from build123d import *

# Parameters (mm, degrees)
PAD_DEPTH          = 3
POCKET_DEPTH       = 3.001
FILLET_R           = 1.5
PAD001_DEPTH       = 8.5
SKETCH004_R        = 2
POCKET001_DEPTH    = 11.501
POCKET002_DEPTH    = 8.5
SKETCH007_R        = 1.5
PAD002_DEPTH       = 2
FILLET001_R        = 1
FILLET002_R        = 2
POLARPATTERN_COUNT = 4


with BuildPart() as part:
    # Sketch → Pad (new body)
    with BuildSketch(Plane.XY):
        with BuildLine():
            Line((0, 0), (28, 0))
            ThreePointArc((23.302356, -15.524181), (26.799869, -8.109687), (28, 0))
            Line((23.302356, -15.524181), (30.833474, -23.0553))
            ThreePointArc((23.0553, -30.833474), (27.223611, -27.223611), (30.833474, -23.0553))
            Line((23.0553, -30.833474), (15.524181, -23.302356))
            ThreePointArc((0, -28), (8.109687, -26.799869), (15.524181, -23.302356))
            Line((0, -28), (0, 0))
        make_face()
    extrude(amount=PAD_DEPTH)

    # Sketch002 (on Face9 of Pad) → Pocket (cut, through all)
    with BuildSketch(Plane.XY.offset(3)):
        Polygon((0, 0), (0, -20), (15.5, -20), (15.5, -15.5), (20, -15.5), (20, 0), align=None)
    extrude(amount=-POCKET_DEPTH, mode=Mode.SUBTRACT)

    # Fillet
    fillet_edges = [part.edges().sort_by_distance(p)[0] for p in [
        (15.5, -15.5, 1.5),
    ]]
    fillet(fillet_edges, radius=FILLET_R)

    # Sketch003 (on Face14 of Fillet) → Pad001 (join)
    with BuildSketch(Plane.XY.offset(3)):
        with BuildLine():
            Line((16.244839, -24.023014), (23.0553, -30.833474))
            ThreePointArc((23.0553, -30.833474), (27.223611, -27.223611), (30.833474, -23.0553))
            Line((30.833474, -23.0553), (24.023014, -16.244839))
            ThreePointArc((16.244839, -24.023014), (20.506097, -20.506097), (24.023014, -16.244839))
        make_face()
    extrude(amount=PAD001_DEPTH)

    # Sketch004 (on Face13 of Pad001) → Pocket001 (cut, through all)
    with BuildSketch(Plane.XY.offset(11.5)):
        with Locations((23.334524, -23.334524)):
            Circle(SKETCH004_R)
    extrude(amount=-POCKET001_DEPTH, mode=Mode.SUBTRACT)

    # Sketch005 (on Face1 of Pocket001) → Pocket002 (cut)
    with BuildSketch(Plane(origin=(0, 0, 0), x_dir=(1, 0, 0), z_dir=(0, 0, -1))):
        with BuildLine():
            ThreePointArc((29.262157, 25.019516), (27.223611, 27.223611), (25.019516, 29.262157))
            Line((25.019516, 29.262157), (18.985551, 23.228191))
            ThreePointArc((23.228191, 18.985551), (21.213203, 21.213203), (18.985551, 23.228191))
            Line((23.228191, 18.985551), (29.262157, 25.019516))
        make_face()
    extrude(amount=-POCKET002_DEPTH, mode=Mode.SUBTRACT)

    # Sketch006 → Groove (revolve, cut)
    with BuildSketch(Plane.YZ):
        Polygon((-38.5, 0), (-38.5, 8.5), (-33, 0), align=None)
    revolve(axis=Axis((0, 0, 0), (0, 0, 1)), mode=Mode.SUBTRACT)

    # Sketch007 (on Face18 of Groove) → Pad002 (join)
    with BuildSketch(Plane.XY.offset(3)):
        with Locations((17, -17)):
            Circle(SKETCH007_R)
    extrude(amount=PAD002_DEPTH)

    # Fillet001
    fillet001_edges = [part.edges().sort_by_distance(p)[0] for p in [
        (20, -15.5, 1.5),
        (15.5, -20, 1.5),
        (18.985551, -23.228191, 4.25),
        (23.228191, -18.985551, 4.25),
    ]]
    fillet(fillet001_edges, radius=FILLET001_R)

    # Fillet002
    fillet002_edges = [part.edges().sort_by_distance(p)[0] for p in [
        (30.833474, -23.0553, 10),
        (23.0553, -30.833474, 10),
    ]]
    fillet(fillet002_edges, radius=FILLET002_R)

    # PolarPattern: part ×4 about axis
    polarpattern_axis = Axis((0, 0, 0), (0, 0, 1))


with BuildPart() as part_1:
    add(part.part)
    for i in range(1, POLARPATTERN_COUNT):
        add(part.part.rotate(polarpattern_axis, i * 360 / POLARPATTERN_COUNT))


solid = part_1.part
For this review, take the finished solid that the model builds, in its own axes (mm). A direction names the side the tool comes from. Coordinates: 2 decimals unless noted, no trailing zeros. Order: outer loops, then holes, each group sorted by start corner. A loop starts at its lowest first (then second) coordinate and runs counter-clockwise, first axis right, second up. Notation, with made-up numbers: (59.25, 10.5) - (88.25, 10.5) arc R31 ccw to (88.25, 37.5) - close; hole circle Ø8 at (20.5, 48.25). An arc over 180 degrees is marked (long way). Answer as CSV lines item,"result". Start each with the question number.
1) To check wall thickness, follow line 1 along Y through (x, z) = (24, 9.5); line 2 along Y through (x, z) = (-21, 1); line 3 along X through (y, z) = (-22.5, 10). State the ranges of each line that lie inside material, in increasing order. Write a range as [from, to].
2) Add section B-B (y = 9). State the section outline as (x, z) points.
3) Add section A-A (z = 9.75). State the section outline as (x, y) points.
4) Draft analysis for pull direction X (two halves, no side actions). For faces 1 (the cylindrical face through (-15.89, 15.99, 3.02)), 2 (the conical face through (27.95, 22.23, 4.19)), 3 (the cylindrical face through (-30.116, 22.775, 9.319)), state which applies: +X half, -X half, draft (parallel to the pull), parting line (faces both ways), or undercut.
5) Add section C-C (x = 2). State the section outline as (y, z) points, then the cut area to 3 significant figures.
6) Machinability: for faces 4 (the flat face through (20, 0, 2)), 5 (the cylindrical face through (21.232, -21.194, 4.19)), 6 (the conical face through (28.14, -21.99, 4.19)), 7 (the cylindrical face through (-27.26, -27.19, 9.98)), 8 (the cylindrical face through (15.99, 15.89, 3.02)), which of the approach directions +Z, -Z, +X, -X, +Y, -Y give a long, thin tool a straight path to every point of the face, cutting with its end or side? Answer none if there is none.
7) Insertion check: P1, Ø2, axis at x = 2, z = 2, coming from the -Y side; P2, Ø0.6, axis at x = -17.5, z = 1, coming from the -Y side; P3, Ø3.5, axis at x = -16.5, y = -16.5, coming from the +Z side; P4, Ø2.5, axis at x = 23.33, y = 23.33, coming from the -Z side. Each pin has a flat end and moves straight along its axis. Give the tip position at first contact, or say it passes through.
Result:
1,line 1,"[-30.01, -25.22], [-21.45, -16.28], [16.28, 21.45], [25.22, 30.01]"
1,line 2,"[-26.29, -25.24], [-21.42, 21.42], [25.24, 26.29]"
1,line 3,"[-30.03, -25.15], [-21.52, -18.3], [18.3, 21.52], [25.15, 30.03]"
2,outline,"(-26.51, 0) - (-20, 0) - (-20, 3) - (-26.51, 3) - close; (20, 0) - (26.51, 0) - (26.51, 3) - (20, 3) - close"
3,outline,"(-29.71, -24.49) arc R38.5 ccw to (-24.49, -29.71) arc R2 ccw to (-21.8, -29.58) - (-16.24, -24.02) arc R29 cw to (-24.02, -16.24) - (-29.58, -21.8) arc R2 ccw to start; (-29.71, 24.49) arc R2 ccw to (-29.58, 21.8) - (-24.02, 16.24) arc R29 cw to (-16.24, 24.02) - (-21.8, 29.58) arc R2 ccw to (-24.49, 29.71) arc R38.5 ccw to start; (16.24, -24.02) - (21.8, -29.58) arc R2 ccw to (24.49, -29.71) arc R38.5 ccw to (29.71, -24.49) arc R2 ccw to (29.58, -21.8) - (24.02, -16.24) arc R29 cw to start; (16.24, 24.02) arc R29 cw to (24.02, 16.24) - (29.58, 21.8) arc R2 ccw to (29.71, 24.49) arc R38.5 ccw to (24.49, 29.71) arc R2 ccw to (21.8, 29.58) - close; hole circle Ø4 at (-23.33, -23.33); hole circle Ø4 at (-23.33, 23.33); hole circle Ø4 at (23.33, -23.33); hole circle Ø4 at (23.33, 23.33)"
4,face 1,"undercut"
4,face 2,"+X half"
4,face 3,"-X half"
5,outline,"(-27.93, 0) - (-20, 0) - (-20, 3) - (-27.93, 3) - close; (20, 0) - (27.93, 0) - (27.93, 3) - (20, 3) - close"
5,area,"47.6 mm^2"
6,face 4,"+Z, -Z"
6,face 5,"-Z"
6,face 6,"-Z, +X, -Y"
6,face 7,"+Z, -Z, -X, -Y"
6,face 8,"+Z"
7,P1,"y = -27.98"
7,P2,"y = -25.58"
7,P3,"z = 5"
7,P4,"through"
